Read the model definition and answer for the solid it produces. Units are mm, in the model's axes. Round coordinates to 2 decimals unless told otherwise and drop trailing zeros. Write each loop counter-clockwise with the first axis right and the second up, starting at its lowest first coordinate (ties: lowest second). Pieces come first, ordered by that corner, then holes. Notation, with made-up numbers: (39.25, 49) -> (50.25, 49) arc R7 ccw to (50.25, 56) -> close; hole circle Ø1 at (6, 71). An arc over 180 degrees is marked (long way). Return JSON: item names as keys, results as strings.
from build123d import *

# Parameters (mm, degrees)
SKETCH1_W           = 45.339
SKETCH1_H           = 355.6
BOSS_EXTRUDE1_DEPTH = 12.7
SKETCH2_W           = 25.4
SKETCH2_H           = 355.6
CUT_EXTRUDE1_DEPTH  = 6.35
SKETCH3_R           = 2.54
CUT_EXTRUDE2_DEPTH  = 7.35


with BuildPart() as part:
    # Sketch1 → Boss-Extrude1 (new body)
    with BuildSketch(Plane.XY):
        with Locations((22.6695, 177.8)):
            Rectangle(SKETCH1_W, SKETCH1_H)
    extrude(amount=BOSS_EXTRUDE1_DEPTH)

    # Sketch2 → Cut-Extrude1 (cut)
    with BuildSketch(Plane(origin=(0, 0, 0), x_dir=(-1, 0, 0), z_dir=(0, 0, -1))):
        with Locations((-22.6695, 177.8)):
            Rectangle(SKETCH2_W, SKETCH2_H)
    extrude(amount=-CUT_EXTRUDE1_DEPTH, mode=Mode.SUBTRACT)

    # Sketch3 → Cut-Extrude2 (cut, through all)
    with BuildSketch(Plane(origin=(0, 0, 6.35), x_dir=(-1, 0, 0), z_dir=(0, 0, -1))):
        with Locations((-22.6695, 19.05)):
            Circle(SKETCH3_R)
        with Locations((-22.6695, 44.45)):
            Circle(SKETCH3_R)
        with Locations((-22.6695, 304.8)):
            Circle(SKETCH3_R)
        with Locations((-22.6695, 279.4)):
            Circle(SKETCH3_R)
        with Locations((-22.6695, 241.3)):
            Circle(SKETCH3_R)
        with Locations((-22.6695, 80.9625)):
            Circle(SKETCH3_R)
    extrude(amount=-CUT_EXTRUDE2_DEPTH, mode=Mode.SUBTRACT)


solid = part.part
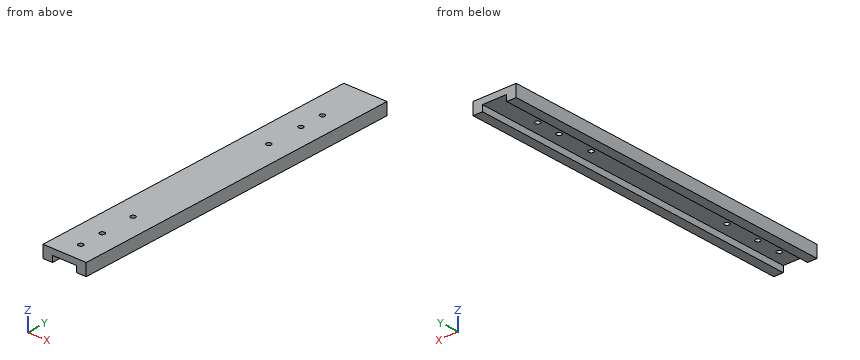
Item 1: A flat-ended cylindrical pin translates along its axis: pin 1 (7.5 mm diameter, centred on x = 20, y = 99, fed in from -Z). Find the tip coordinate at first contact, or state that the pin passes through.
Worked answers:
{"pin 1": "stops at z = 6.35"}
Item 2: Straight lines are drawn through the part: L1, parallel to X at y = 298, z = 2; L2, parallel to X at y = 279.4, z = 9.5; L3, parallel to Z at x = 17, y = 65. For each, find the intervals that lie inside material, in ascending order. Write a range as [from, to].
Worked answers:
{"L1": "x = [0, 9.97], [35.37, 45.34]", "L2": "x = [0, 20.13], [25.21, 45.34]", "L3": "z = [6.35, 12.7]"}
Item 3: Section B-B (x = 13) is taken. Give the vertices of the cut face in (y, z), then the cut area to 3 significant figures.
Worked answers:
{"outline": "(0, 6.35) -> (355.6, 6.35) -> (355.6, 12.7) -> (0, 12.7) -> close", "area": "2,260 mm2"}
Item 4: Section A-A (y = 26) is taken. Give the vertices of the cut face in (x, z).
Worked answers:
{"outline": "(0, 0) -> (9.97, 0) -> (9.97, 6.35) -> (35.37, 6.35) -> (35.37, 0) -> (45.34, 0) -> (45.34, 12.7) -> (0, 12.7) -> close"}
